Drawing for the job (mm, zero at the part's lowest x, y, z). Give positions to 0.01 mm unless a question says otherwise; leave off trailing zeros. Order: outer loops, then holes, each group sorted by start corner. A loop starts at its lowest first (then second) coordinate and runs counter-clockwise, first axis right, second up. Notation, with made-up numbers: (63, 3.25) - (84, 3.25) arc R17 cw to (84, 33.25) - close; hole circle Ø10 at (31.25, 19.25). An arc over 180 degrees is marked (long way). Use a Markdown table: item, result. Add a question column.
(1) Slice it at C-C (z = 2.85). Write the cut outline in (x, y).
(2) Flat gauge pins, fed straight in: pin 1 (1.6 mm diameter, centred on x = 34, y = 1, fed in from +Z); pin 2 (13.5 mm diameter, centred on x = 60.55, y = 53.05, fed in from +Z); pin 3 (0.6 mm diameter, centred on x = 43, z = 5.5, fed in from -Y); pin 4 (3 mm diameter, centred on x = 52, y = 58.5, fed in from -Z). Where does each tip first touch, or does it go through?
(3) Mould opens along X. For the marked faces 1 and 2 say: +X half, -X half, draft (parallel to the pull), parting line (faces both ways), or undercut.
(4) Wall check: line 1 (Y direction, x = 60.55, z = 4.05); line 2 (X direction, y = 53.05, z = 4.05); line 3 (X direction, y = 35.5, z = 5.4). Give the ranges that are in metal, low to high.
(5) Slice it at B-B (y = 35). Write the cut outline in (x, z).
(6) Slice it at A-A (x = 42). Write the cut outline in (y, z).
(7) Slice it at D-D (x = 60.55). Count the separate pieces of the cut face and the enclosed holes in it.
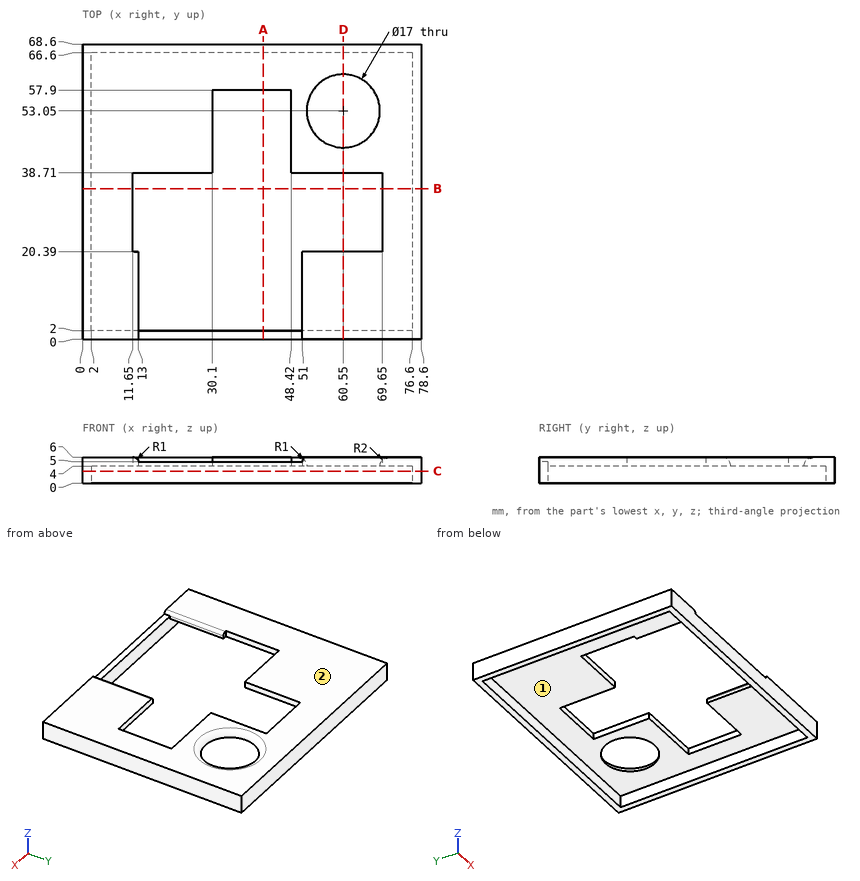
Solution:
| question | item | result |
|---|---|---|
| 1 | outline | (0, 0) - (78.6, 0) - (78.6, 68.6) - (0, 68.6) - close; hole (2, 2) - (76.6, 2) - (76.6, 66.6) - (2, 66.6) - close |
| 2 | pin 1 | z = 5 |
| 2 | pin 2 | through |
| 2 | pin 3 | y = 57.9 |
| 2 | pin 4 | z = 4 |
| 3 | face 1 | undercut |
| 3 | face 2 | draft |
| 4 | line 1 | 0 to 20.39, 38.71 to 44.55, 61.55 to 68.6 |
| 4 | line 2 | 0 to 30.1, 48.42 to 52.05, 69.05 to 78.6 |
| 4 | line 3 | 0 to 11.65, 69.65 to 78.6 |
| 5 | outline | (0, 0) - (2, 0) - (2, 4) - (11.65, 4) - (11.65, 6) - (0, 6) - close; (69.65, 4) - (76.6, 4) - (76.6, 0) - (78.6, 0) - (78.6, 6) - (69.65, 6) - close |
| 6 | outline | (0, 0) - (2, 0) - (2, 5) - (0, 5) - close; (57.9, 4) - (66.6, 4) - (66.6, 0) - (68.6, 0) - (68.6, 6) - (57.9, 6) - close |
| 7 | separate pieces | 3 |
| 7 | enclosed holes | 0 |
